Source: CAD feature listing. Evaluate the final solid. Frame: model axes, mm. A direction names the side the tool comes from. Give positions to 0.01 mm unless a question says otherwise; leave off trailing zeros. Order: outer loops, then holes, each group sorted by start corner. A loop starts at its lowest first (then second) coordinate and runs counter-clockwise, first axis right, second up. Notation, with made-up numbers: M 37.5,17 L 81.5,17 A28 ccw 81.5,36 Z; hole C 69,81.5 d4. An arc over 180 degrees is marked long. Return JSON: item names as keys, results as strings.
from build123d import *

# Parameters (mm, degrees)
F0_W           = 100
F0_H           = 60
F1_DEPTH       = 25
F2_T           = -2.5
F3_R           = 5
F4_R           = 5
F5_R           = 3.5
F6_DEPTH       = 25
F7_R           = 1.24999
F8_R           = 5
F8_R_2         = 1
F9_DEPTH       = 25
F10_DEPTH      = 1
F10_DEPTH_BACK = 1
F11_R          = 5
F12_DEPTH      = 25
F13_R          = 5
F14_DEPTH      = 25
F15_R          = 5
F16_DEPTH      = 25
F17_R          = 6.25
F18_DEPTH      = 10


# Not quite as in the source:
# - a fillet or chamfer is up to 0.001 mm smaller than in the source, because OpenCascade refuses the exact size


with BuildPart() as f1:
    # F0 (on Top) → F1 (new body)
    with BuildSketch(Plane.XY):
        with Locations((23.0550479144, 14.1446392238)):
            Rectangle(F0_W, F0_H)
    extrude(amount=F1_DEPTH)

    # F2
    f2_openings = [f1.faces().sort_by_distance(p)[0] for p in [
        (23.055048, 14.144639, 25),
    ]]
    offset(amount=F2_T, openings=f2_openings)

    # F3
    f3_edges = [f1.edges().sort_by_distance(p)[0] for p in [
        (-26.944952, 44.144639, 12.5),
        (-26.944952, -15.855361, 12.5),
        (73.055048, -15.855361, 12.5),
        (73.055048, 44.144639, 12.5),
    ]]
    fillet(f3_edges, radius=F3_R)

    # F4
    f4_edges = [f1.edges().sort_by_distance(p)[0] for p in [
        (70.555048, -13.355361, 13.75),
        (-24.444952, 41.644639, 13.75),
        (-24.444952, -13.355361, 13.75),
        (70.555048, 41.644639, 13.75),
    ]]
    fillet(f4_edges, radius=F4_R)

    # F5 (on face) → F6 (cut)
    with BuildSketch(Plane.XY.offset(2.5)):
        with Locations((26.5453665042, 10.6446392238)):
            Circle(F5_R)
    extrude(amount=-F6_DEPTH, mode=Mode.SUBTRACT)

    # F7 (radius 1.25 in the source; OpenCascade refuses exactly that, so slightly less here)
    f7_edges = [f1.edges().sort_by_distance(p)[0] for p in [
        (23.045367, 10.644639, 0),
        (23.045367, 10.644639, 2.5),
    ]]
    fillet(f7_edges, radius=F7_R)

    # F8 (on face) → F9 (join)
    with BuildSketch(Plane.XY):
        with Locations((-19.9449520856, 37.1446392238)):
            Circle(F8_R)
        with Locations((-19.9449520856, 37.1446392238)):
            Circle(F8_R_2, mode=Mode.SUBTRACT)
    extrude(amount=F9_DEPTH)

    # F10 (cut, two sides): a face of the model
    f10_faces = [f1.faces().sort_by_distance(p)[0] for p in [
        (-19.9449520856, 37.1446392238, 2.5),
    ]]
    extrude(f10_faces, amount=-F10_DEPTH, mode=Mode.SUBTRACT)
    extrude(f10_faces, amount=F10_DEPTH_BACK, mode=Mode.SUBTRACT)

    # F11 (on face) → F12 (join)
    with BuildSketch(Plane.XY):
        with Locations((66.0550479144, 37.1446392238)):
            Circle(F11_R)
    extrude(amount=F12_DEPTH)

    # F13 (on face) → F14 (join)
    with BuildSketch(Plane.XY):
        with Locations((-19.9449520856, -8.8553607762)):
            Circle(F13_R)
    extrude(amount=F14_DEPTH)

    # F15 (on face) → F16 (join)
    with BuildSketch(Plane.XY):
        with Locations((66.0550479144, -8.8553607762)):
            Circle(F15_R)
    extrude(amount=F16_DEPTH)

    # F17 (on face) → F18 (cut)
    with BuildSketch(Plane(origin=(0, 44.1446392238, 0), x_dir=(-1, 0, 0), z_dir=(0, 1, 0))):
        with Locations((-23.0550479144, 12.8674265233)):
            Circle(F17_R)
    extrude(amount=-F18_DEPTH, mode=Mode.SUBTRACT)


solid = f1.part
1. Ray query, probe 1 along X at (y, z) = (37, 7.25); probe 2 along X at (y, z) = (-2, 14.25); probe 3 along Y at (x, z) = (31, 5.25). Return the intervals inside material, ascending.
Evaluation:
{"probe 1": "x = -26.94 to -20.93, -18.96 to -14.95, 61.06 to 73.06", "probe 2": "x = -26.94 to -24.44, 70.56 to 73.06", "probe 3": "y = -15.86 to -13.36, 41.64 to 44.14"}
2. Section query C-C (z = 23.75). Return loops of the section in (x, y), then the cut area to 3 significant figures.
Evaluation:
{"outline": "M -26.94,-10.86 A5 ccw -21.94,-15.86 L 68.06,-15.86 A5 ccw 73.06,-10.86 L 73.06,39.14 A5 ccw 68.06,44.14 L -21.94,44.14 A5 ccw -26.94,39.14 Z; hole M -24.44,-6.68 A5 cw long -17.77,-13.36 L 63.88,-13.36 A5 cw long 70.56,-6.68 L 70.56,34.97 A5 cw long 63.88,41.64 L -17.77,41.64 A5 cw long -24.44,34.97 Z; hole C -19.94,37.14 d2", "area": "1,060 mm^2"}
3. Draft query along Y for faces 4 (the face through (22, 44.145, 4)), 5 (the face through (22, -15.855, 12)), 6 (the face through (-16.316, -5.415, 13.592)). Return one class per face: pulls with the +Y half, pulls with the -Y half, needs draft (parallel to the pull), parting line crosses it, or undercut.
Evaluation:
{"face 4": "pulls with the +Y half", "face 5": "pulls with the -Y half", "face 6": "undercut"}
4. Section query D-D (z = 15.75). Return loops of the section in (x, y).
Evaluation:
{"outline": "M -26.94,-10.86 A5 ccw -21.94,-15.86 L 68.06,-15.86 A5 ccw 73.06,-10.86 L 73.06,39.14 A5 ccw 68.06,44.14 L 28.6,44.14 L 28.6,41.64 L 63.88,41.64 A5 ccw long 70.56,34.97 L 70.56,-6.68 A5 ccw long 63.88,-13.36 L -17.77,-13.36 A5 ccw long -24.44,-6.68 L -24.44,34.97 A5 ccw long -17.77,41.64 L 17.51,41.64 L 17.51,44.14 L -21.94,44.14 A5 ccw -26.94,39.14 Z; hole C -19.94,37.14 d2"}
5. Section query A-A (x = 12.5). Return loops of the section in (y, z).
Evaluation:
{"outline": "M -15.86,0 L 44.14,0 L 44.14,25 L 41.64,25 L 41.64,2.5 L -13.36,2.5 L -13.36,25 L -15.86,25 Z"}
6. Set-up query: faces 1 (the face through (71.63, 42.64, 12.68)), 2 (the face through (17.282, 42.912, 10.474)), 3 (the face through (22, 15, 2.5)). Return all of +Z, -Z, +X, -X, +Y, -Y with unobstructed straight access to the full face (end or side cutting, diameter ignored); none if empty.
Evaluation:
{"face 1": "+Z, -Z, +X, +Y", "face 2": "+Y", "face 3": "+Z"}
7. Section query B-B (z = 11.25). Return loops of the section in (x, y).
Evaluation:
{"outline": "M -26.94,-10.86 A5 ccw -21.94,-15.86 L 68.06,-15.86 A5 ccw 73.06,-10.86 L 73.06,39.14 A5 ccw 68.06,44.14 L 29.09,44.14 L 29.09,41.64 L 63.88,41.64 A5 ccw long 70.56,34.97 L 70.56,-6.68 A5 ccw long 63.88,-13.36 L -17.77,-13.36 A5 ccw long -24.44,-6.68 L -24.44,34.97 A5 ccw long -17.77,41.64 L 17.02,41.64 L 17.02,44.14 L -21.94,44.14 A5 ccw -26.94,39.14 Z; hole C -19.94,37.14 d2"}
8. First-contact query: pin 1 (8 mm diameter, centred on x = 26.55, y = 10.64, fed in from +Z). Flat tip, straight axial feed; report the tip coordinate or a pass-through.
Evaluation:
{"pin 1": "stops at z = 2.25"}
